Here's how the part is built. I have some questions about the finished solid (model axes, mm). A direction names the side the tool comes from. Coordinates: 2 decimals unless noted, no trailing zeros. Loops run counter-clockwise (first coordinate to the right, second up) from the corner with the lowest first, then second, coordinate; pieces in that order, holes last. Notation, with made-up numbers: (88.5, 7) -> (118.5, 7) arc R34 ccw to (118.5, 42) -> close; hole circle Ø1 at (-14.75, 6.5). An arc over 180 degrees is marked (long way). Answer as a JSON object with one key per item and string values. Group by question number.
1) I'm going to push flat-ended pins straight in: pin 1 (1.5 mm diameter, centred on x = 1.5, y = 8.5, fed in from +Z); pin 2 (1.5 mm diameter, centred on y = 5.5, z = 1, fed in from +X); pin 3 (3 mm diameter, centred on x = -2, z = 3.5, fed in from +Y). Where does each tip first touch, or does it pass through?
2) I want a section at D-D (y = 8.5). Write out the boundary of the cut face in (x, z), then the cut area to 3 significant figures.
3) If we mould it in two halves opening along X, with no side actions, what happens to faces 4 (the flat face through (-5.1, 2, 3)), 5 (the flat face through (0.8, 1.1, 2.9)), 6 (the flat face through (0.55, 0.5, 2.9)), 7 (the flat face through (-2.5, 0, 2.9))? For each: +X half, -X half, draft (parallel to the pull), parting line (faces both ways), or undercut.
4) Which directions (+Z, -Z, +X, -X, +Y, -Y) give clear straight access to the entire face, cutting with the end or side of a thin tool? Please do faces 1 (the flat face through (1, 6, 1)), 2 (the flat face through (2.5, 0, 2.9)), 3 (the flat face through (-4.53, 0.5, 2.9)).
5) I want a section at A-A (z = 5.15). Write out the boundary of the cut face in (x, y), then the cut area to 3 significant figures.
6) I want a section at C-C (x = 4.75). Write out the boundary of the cut face in (y, z), then the cut area to 3 significant figures.
7) I need wall thicknesses on probe 1 along X at (y, z) = (0.5, 4.8); probe 2 along Z at (x, y) = (1, 2.5); probe 3 along X at (y, z) = (9.5, 0.55). Which ranges of each line are inside material? Lowest first, please. Write a range as [from, to].
```python
from build123d import *

# Parameters (mm, degrees)
AUFSATZ_LINEAR_AUSTRAGEN1_DEPTH = 5.8
SKIZZE1_3_W                     = 4.5
SKIZZE1_3_H                     = 1.8
AUFSATZ_LINEAR_AUSTRAGEN2_DEPTH = 0.8
SKIZZE1_4_W                     = 4.5
SKIZZE1_4_H                     = 1.8
AUFSATZ_LINEAR_AUSTRAGEN3_DEPTH = 1
FASE1_SIZE                      = 0.2
VERRUNDUNG1_START               = -2
VERRUNDUNG1_DEPTH               = 7
VERRUNDUNG1_START_2             = 4
VERRUNDUNG1_2_DEPTH             = 4
SKIZZE3_W                       = 0.6
SKIZZE3_H                       = 0.6
SCHNITT_LINEAR_AUSTRAGEN1_DEPTH = 12.119802157
FASE2_SIZE                      = 0.42


with BuildPart() as part:
    # Skizze1 → Aufsatz-Linear austragen1 (new body)
    with BuildSketch(Plane.XY):
        Polygon((-1.99, 1.1), (-0.55, 1.1), (-0.55, 0), (0.55, 0), (0.55, 1.1), (1.99, 1.1), (1.99, 0), (3.09, 0), (3.09, 1.1), (4.53, 1.1), (4.53, 0), (5.1, 0), (5.1, 3.4), (3.8, 3.4), (-1.2, 3.4), (-5.1, 3.4), (-5.1, 0), (-4.53, 0), (-4.53, 1.1), (-3.09, 1.1), (-3.09, 0), (-1.99, 0), align=None)
    extrude(amount=AUFSATZ_LINEAR_AUSTRAGEN1_DEPTH)

    # Skizze1<3> → Aufsatz-Linear austragen2 (add)
    # profile 1 of 2: a face of its own
    with BuildSketch(Plane.XY):
        with BuildLine():
            Line((-1.2, 10.6), (-1.2, 3.4))
            Line((-1.2, 3.4), (3.8, 3.4))
            Line((3.8, 3.4), (3.8, 10.6))
            ThreePointArc((3.8, 10.6), (3.565685425, 11.165685425), (3, 11.4))
            Line((3, 11.4), (-0.4, 11.4))
            ThreePointArc((-0.4, 11.4), (-0.965685425, 11.165685425), (-1.2, 10.6))
        make_face()
        with Locations((1.3, 6.1)):
            Rectangle(SKIZZE1_3_W, SKIZZE1_3_H, mode=Mode.SUBTRACT)
    # profile 2 of 2: a face of its own
    with BuildSketch(Plane.XY):
        with Locations((1.3, 6.1)):
            Rectangle(SKIZZE1_3_W, SKIZZE1_3_H)
    extrude(amount=AUFSATZ_LINEAR_AUSTRAGEN2_DEPTH)

    # Skizze1<4> → Aufsatz-Linear austragen3 (add)
    with BuildSketch(Plane.XY):
        with Locations((1.3, 6.1)):
            Rectangle(SKIZZE1_4_W, SKIZZE1_4_H)
    extrude(amount=AUFSATZ_LINEAR_AUSTRAGEN3_DEPTH)

    # Fase1
    fase1_edges = [part.edges().sort_by_distance(p)[0] for p in [
        (-0.95, 6.1, 0.8),
        (1.3, 5.2, 0.8),
        (3.55, 6.1, 0.8),
        (1.3, 7, 0.8),
    ]]
    chamfer(fase1_edges, length=FASE1_SIZE - 0.0001)  # a hair under: the kernel refuses the full size

    # Verrundung1: read off the stored shape, not the designer's step
    # Verrundung1 outline → Verrundung1 (cut)
    with BuildSketch(Plane.YZ.offset(VERRUNDUNG1_START)):
        with BuildLine():
            ThreePointArc((5, 0.8), (5.283772234, 0.948683298), (5.6, 1))
            Line((5.6, 1), (5.2, 1))
            Line((5.2, 1), (5, 0.8))
        make_face()
        with BuildLine():
            ThreePointArc((6.6, 1), (6.916227766, 0.948683298), (7.2, 0.8))
            Line((7.2, 0.8), (7, 1))
            Line((7, 1), (6.6, 1))
        make_face()
    extrude(amount=VERRUNDUNG1_DEPTH, mode=Mode.SUBTRACT)

    # Verrundung1 2 outline → Verrundung1 2 (cut)
    with BuildSketch(Plane(origin=(0, 0, 0), x_dir=(1, 0, 0), z_dir=(0, 1, 0)).offset(VERRUNDUNG1_START_2)):
        with BuildLine():
            Line((-0.95, -1), (-0.55, -1))
            ThreePointArc((-0.55, -1), (-0.866227766, -0.948683298), (-1.15, -0.8))
            Line((-1.15, -0.8), (-0.95, -1))
        make_face()
        with BuildLine():
            ThreePointArc((3.75, -0.8), (3.466227766, -0.948683298), (3.15, -1))
            Line((3.15, -1), (3.55, -1))
            Line((3.55, -1), (3.75, -0.8))
        make_face()
    extrude(amount=VERRUNDUNG1_2_DEPTH, mode=Mode.SUBTRACT)

    # Skizze3 → Schnitt-Linear austragen1 (cut, through all)
    with BuildSketch(Plane(origin=(0, 3.4, 0), x_dir=(1, 0, 0), z_dir=(0, 1, 0))):
        with Locations((1.27, -2.6)):
            Rectangle(SKIZZE3_W, SKIZZE3_H)
        with Locations((-1.27, -2.6)):
            Rectangle(SKIZZE3_W, SKIZZE3_H)
        with Locations((-3.81, -2.6)):
            Rectangle(SKIZZE3_W, SKIZZE3_H)
        with Locations((3.81, -2.6)):
            Rectangle(SKIZZE3_W, SKIZZE3_H)
    extrude(amount=-SCHNITT_LINEAR_AUSTRAGEN1_DEPTH, mode=Mode.SUBTRACT)

    # Fase2
    fase2_edges = [part.edges().sort_by_distance(p)[0] for p in [
        (3.81, 3.4, 2.3),
        (3.51, 3.4, 2.6),
        (3.81, 3.4, 2.9),
        (4.11, 3.4, 2.6),
        (1.27, 3.4, 2.3),
        (0.97, 3.4, 2.6),
        (1.27, 3.4, 2.9),
        (1.57, 3.4, 2.6),
        (-3.51, 3.4, 2.6),
        (-3.81, 3.4, 2.3),
        (-4.11, 3.4, 2.6),
        (-3.81, 3.4, 2.9),
        (-0.97, 3.4, 2.6),
        (-1.27, 3.4, 2.3),
        (-1.57, 3.4, 2.6),
        (-1.27, 3.4, 2.9),
    ]]
    chamfer(fase2_edges, length=FASE2_SIZE)


solid = part.part
```
Determined:
{
 "1": {"pin 1": "z = 0.8", "pin 2": "x = 3.8", "pin 3": "y = 3.4"},
 "2": {"outline": "(-1.2, 0) -> (3.8, 0) -> (3.8, 0.8) -> (-1.2, 0.8) -> close", "area": "4.00 mm^2"},
 "3": {"face 4": "-X half", "face 5": "undercut", "face 6": "undercut", "face 7": "draft"},
 "4": {"face 1": "+Z, +X, -X, +Y", "face 2": "+Z, -Z, +X, -X, -Y", "face 3": "+Z, -Z, -Y"},
 "5": {"outline": "(-5.1, 0) -> (-4.53, 0) -> (-4.53, 1.1) -> (-3.09, 1.1) -> (-3.09, 0) -> (-1.99, 0) -> (-1.99, 1.1) -> (-0.55, 1.1) -> (-0.55, 0) -> (0.55, 0) -> (0.55, 1.1) -> (1.99, 1.1) -> (1.99, 0) -> (3.09, 0) -> (3.09, 1.1) -> (4.53, 1.1) -> (4.53, 0) -> (5.1, 0) -> (5.1, 3.4) -> (-5.1, 3.4) -> close", "area": "28.3 mm^2"},
 "6": {"outline": "(0, 0) -> (3.4, 0) -> (3.4, 5.8) -> (0, 5.8) -> close", "area": "19.7 mm^2"},
 "7": {"probe 1": "[-5.1, -4.53], [-3.09, -1.99], [-0.55, 0.55], [1.99, 3.09], [4.53, 5.1]", "probe 2": "[0, 2.3], [2.9, 5.8]", "probe 3": "[-1.2, 3.8]"}
}
